from build123d import *

# Parameters (mm, degrees)
SKETCH1_W                                       = 63.5
SKETCH1_H                                       = 63.5
BOSS_EXTRUDE1_DEPTH                             = 6.35
F_6_32_TAPPED_HOLE1_D                           = 2.7051
SKETCH4_R                                       = 21.0439
SKETCH4_R_2                                     = 16.7767
CUT_EXTRUDE1_DEPTH                              = 2.0066
SKETCH5_R                                       = 16.7767
BOSS_EXTRUDE2_DEPTH                             = 0.508
CSK_FOR_M4_FLAT_HEAD_MACHINE_SCREW1_D           = 4.5
CSK_FOR_M4_FLAT_HEAD_MACHINE_SCREW1_CSINK_D     = 9.4
CSK_FOR_M4_FLAT_HEAD_MACHINE_SCREW1_CSINK_ANGLE = 90
CUT_EXTRUDE2_DEPTH                              = 7.858


with BuildPart() as part:
    # Sketch1 → Boss-Extrude1 (new body)
    with BuildSketch(Plane.XY):
        Rectangle(SKETCH1_W, SKETCH1_H)
    extrude(amount=BOSS_EXTRUDE1_DEPTH)

    # #6-32 Tapped Hole1 (through all)
    with Locations(Plane(origin=(0, 0, 0), x_dir=(-1, 0, 0), z_dir=(0, 0, -1))):
        with Locations((20.6375, -20.6375), (-20.6375, -20.6375), (-20.6375, 20.6375), (20.6375, 20.6375)):
            Hole(F_6_32_TAPPED_HOLE1_D / 2)

    # Sketch4 → Cut-Extrude1 (cut)
    with BuildSketch(Plane.XY.offset(6.35)):
        with Locations((0, 6.076865153)):
            Circle(SKETCH4_R)
        with Locations((0, 6.076865153)):
            Circle(SKETCH4_R_2, mode=Mode.SUBTRACT)
    extrude(amount=-CUT_EXTRUDE1_DEPTH, mode=Mode.SUBTRACT)

    # Sketch5 → Boss-Extrude2 (add)
    with BuildSketch(Plane.XY.offset(6.35)):
        with Locations((0, 6.076865153)):
            Circle(SKETCH5_R)
    extrude(amount=BOSS_EXTRUDE2_DEPTH)

    # CSK for M4 Flat Head Machine Screw1 (through all)
    with Locations(Plane(origin=(0, 0, 0), x_dir=(-1, 0, 0), z_dir=(0, 0, -1))):
        with Locations((-25.691176831, 6.076865153), (25.691176831, 6.076865153)):
            CounterSinkHole(CSK_FOR_M4_FLAT_HEAD_MACHINE_SCREW1_D / 2, CSK_FOR_M4_FLAT_HEAD_MACHINE_SCREW1_CSINK_D / 2, counter_sink_angle=CSK_FOR_M4_FLAT_HEAD_MACHINE_SCREW1_CSINK_ANGLE)

    # Sketch9 → Cut-Extrude2 (cut, through all)
    with BuildSketch(Plane(origin=(0, 0, 0), x_dir=(-1, 0, 0), z_dir=(0, 0, -1))):
        with BuildLine():
            Line((9.525, 11.1125), (9.525, -5.754710044))
            ThreePointArc((9.525, -5.754710044), (0, -9.112334847), (-9.525, -5.754710044))
            Line((-9.525, -5.754710044), (-9.525, 11.1125))
            ThreePointArc((-9.525, 11.1125), (-8.130096045, 14.480096045), (-4.7625, 15.875))
            Line((-4.7625, 15.875), (4.7625, 15.875))
            ThreePointArc((4.7625, 15.875), (8.130096045, 14.480096045), (9.525, 11.1125))
        make_face()
    extrude(amount=-CUT_EXTRUDE2_DEPTH, mode=Mode.SUBTRACT)


solid = part.part
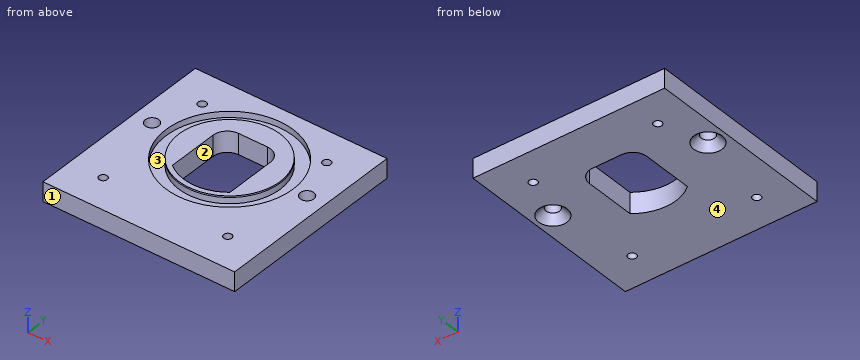
For this review, take the finished solid that the model builds, in its own axes (mm). Face numbers are marked on the shaded views. A direction names the side the tool comes from. Give positions to 0.01 mm unless a question says otherwise; leave off trailing zeros. Order: outer loops, then holes, each group sorted by start corner. A loop starts at its lowest first (then second) coordinate and runs counter-clockwise, first axis right, second up. Notation, with made-up numbers: (29, 67.25) - (84, 67.25) arc R21 ccw to (84, 99.25) - close; hole circle Ø8 at (21.5, 45). An arc over 180 degrees is marked (long way). Answer as a JSON object with one key per item and string values. Group by question number.
Item 1: Take a section at B-B on y = -3.5. Give the boundary of the cut face in (x, z) (3 decimals).
Item 2: Wall thickness on line 1 along X through (y, z) = (20.5, 2); line 2 along Y through (x, z) = (-3, 4.5) (3 decimals); line 3 along Y through (x, z) = (-20, 0.75): over which ranges is each line inside the solid? List them lowest first.
Item 3: Take a section at D-D on y = -13. Give the boundary of the cut face in (x, z), and give its area (3 significant figures).
Item 4: Take a section at A-A on x = 0. Give the boundary of the cut face in (y, z) (3 decimals).
Item 5: Clearance check with a flat-ended pin moving along its axis: pin 1 Ø3.5 at (x, y) = (20.64, 20.64) entering from +Z. State where the tip first meets the part, or that it passes through.
Item 6: Draft analysis for pull direction X (two halves, no side actions). For the marked faces 3 and 4, state which applies: pulls with the +X half, pulls with the -X half, needs draft (parallel to the pull), parting line crosses it, or undercut.
Item 7: Take a section at C-C on x = 15.5. Give the boundary of the cut face in (y, z).
Item 8: Machinability: for the marked faces 1 and 2, which of the approach directions +Z, -Z, +X, -X, +Y, -Y give a long, thin tool a straight path to every point of the face, cutting with its end or side? Answer none if there is none.
Reported:
{
 "1": {"outline": "(-31.75, 0) - (-9.525, 0) - (-9.525, 6.858) - (-13.775, 6.858) - (-13.775, 4.343) - (-18.738, 4.343) - (-18.738, 6.35) - (-31.75, 6.35) - close; (9.525, 0) - (31.75, 0) - (31.75, 6.35) - (18.738, 6.35) - (18.738, 4.343) - (13.775, 4.343) - (13.775, 6.858) - (9.525, 6.858) - close"},
 "2": {"line 1": "-31.75 to -21.98, -19.29 to 19.29, 21.98 to 31.75", "line 2": "-31.75 to -14.752, -10.429 to -8.813, 15.875 to 22.583, 26.906 to 31.75", "line 3": "-31.75 to -21.83, -19.44 to 19.44, 21.83 to 31.75"},
 "3": {"outline": "(-31.75, 0) - (31.75, 0) - (31.75, 6.35) - (8.88, 6.35) - (8.88, 4.34) - (-8.88, 4.34) - (-8.88, 6.35) - (-31.75, 6.35) - close", "area": "368 mm^2"},
 "4": {"outline": "(-31.75, 0) - (-9.112, 0) - (-9.112, 6.858) - (-10.7, 6.858) - (-10.7, 4.343) - (-14.967, 4.343) - (-14.967, 6.35) - (-31.75, 6.35) - close; (15.875, 0) - (31.75, 0) - (31.75, 6.35) - (27.121, 6.35) - (27.121, 4.343) - (22.854, 4.343) - (22.854, 6.858) - (15.875, 6.858) - close"},
 "5": {"pin 1": "z = 6.35"},
 "6": {"face 3": "undercut", "face 4": "needs draft"},
 "7": {"outline": "(-31.75, 0) - (31.75, 0) - (31.75, 6.35) - (20.31, 6.35) - (20.31, 4.34) - (12.5, 4.34) - (12.5, 6.86) - (-0.34, 6.86) - (-0.34, 4.34) - (-8.16, 4.34) - (-8.16, 6.35) - (-31.75, 6.35) - close"},
 "8": {"face 1": "+Z, -Z, +X, -X, -Y", "face 2": "+Z, -Z"}
}
